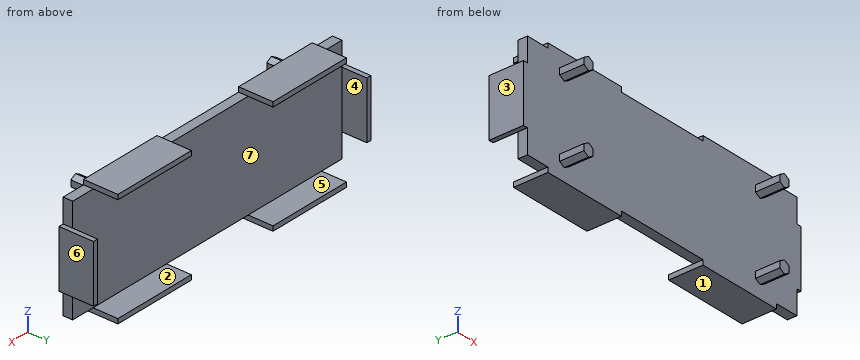
```python
from build123d import *

# Parameters (mm, degrees)
SKETCH1_W           = 165
SKETCH1_H           = 55
BOSS_EXTRUDE1_DEPTH = 5
SKETCH2_W           = 2.5
SKETCH2_H           = 30
BOSS_EXTRUDE2_DEPTH = 18
SKETCH3_W           = 45
SKETCH3_H           = 2.5
BOSS_EXTRUDE3_DEPTH = 18
BOSS_EXTRUDE4_DEPTH = 12.75


with BuildPart() as part:
    # Sketch1 → Boss-Extrude1 (new body)
    with BuildSketch(Plane(origin=(0, 0, 0), x_dir=(1, 0, 0), z_dir=(0, 1, 0))):
        with Locations((82.5, 27.5)):
            Rectangle(SKETCH1_W, SKETCH1_H)
    extrude(amount=BOSS_EXTRUDE1_DEPTH)

    # Sketch2 → Boss-Extrude2 (add)
    with BuildSketch(Plane(origin=(0, 0, 0), x_dir=(1, 0, 0), z_dir=(0, 1, 0))):
        with Locations((166.25, 27.5)):
            Rectangle(SKETCH2_W, SKETCH2_H)
        with Locations((-1.25, 27.5)):
            Rectangle(SKETCH2_W, SKETCH2_H)
    extrude(amount=BOSS_EXTRUDE2_DEPTH)

    # Sketch3 → Boss-Extrude3 (add)
    with BuildSketch(Plane(origin=(0, 0, 0), x_dir=(1, 0, 0), z_dir=(0, 1, 0))):
        with Locations((130, 56.25)):
            Rectangle(SKETCH3_W, SKETCH3_H)
        with Locations((35, 56.25)):
            Rectangle(SKETCH3_W, SKETCH3_H)
        with Locations((130, -1.25)):
            Rectangle(SKETCH3_W, SKETCH3_H)
        with Locations((35, -1.25)):
            Rectangle(SKETCH3_W, SKETCH3_H)
    extrude(amount=BOSS_EXTRUDE3_DEPTH)

    # Sketch4 → Boss-Extrude4 (add)
    with BuildSketch(Plane.XZ):
        Polygon((139.65, -5.854551733), (139.65, -9.145448267), (142.5, -10.790896534), (145.35, -9.145448267), (145.35, -5.854551733), (142.5, -4.209103466), align=None)
        Polygon((22.5, -10.790896534), (25.35, -9.145448267), (25.35, -5.854551733), (22.5, -4.209103466), (19.65, -5.854551733), (19.65, -9.145448267), align=None)
        Polygon((22.5, -50.790896534), (25.35, -49.145448267), (25.35, -45.854551733), (22.5, -44.209103466), (19.65, -45.854551733), (19.65, -49.145448267), align=None)
        Polygon((145.35, -49.145448267), (145.35, -45.854551733), (142.5, -44.209103466), (139.65, -45.854551733), (139.65, -49.145448267), (142.5, -50.790896534), align=None)
    extrude(amount=BOSS_EXTRUDE4_DEPTH)


solid = part.part
```
Part model, mm, in its own coordinate system. Face numbers are marked on the shaded views. A direction names the side the tool comes from. Give positions to 0.01 mm unless a question says otherwise; leave off trailing zeros. Order: outer loops, then holes, each group sorted by start corner. A loop starts at its lowest first (then second) coordinate and runs counter-clockwise, first axis right, second up. Notation, with made-up numbers: (53.5, 15) - (72.5, 15) arc R17 ccw to (72.5, 27) - close; hole circle Ø11 at (9, 70.5). An arc over 180 degrees is marked (long way). Use one line per item in the form item = value.
Item 1: Slice it at D-D on x = 52.5. Give the cut face in (y, z).
Solution:
outline = (0, -57.5) - (18, -57.5) - (18, -55) - (5, -55) - (5, 0) - (18, 0) - (18, 2.5) - (0, 2.5) - close
Item 2: Slice it at B-B on y = -6. Give the cut face in (x, z).
Solution:
outline = (19.65, -49.15) - (22.5, -50.79) - (25.35, -49.15) - (25.35, -45.85) - (22.5, -44.21) - (19.65, -45.85) - close; (19.65, -9.15) - (22.5, -10.79) - (25.35, -9.15) - (25.35, -5.85) - (22.5, -4.21) - (19.65, -5.85) - close; (139.65, -49.15) - (142.5, -50.79) - (145.35, -49.15) - (145.35, -45.85) - (142.5, -44.21) - (139.65, -45.85) - close; (139.65, -9.15) - (142.5, -10.79) - (145.35, -9.15) - (145.35, -5.85) - (142.5, -4.21) - (139.65, -5.85) - close
Item 3: Slice it at C-C on z = -25. Give the cut face in (x, y).
Solution:
outline = (-2.5, 0) - (167.5, 0) - (167.5, 18) - (165, 18) - (165, 5) - (0, 5) - (0, 18) - (-2.5, 18) - close
Item 4: Two-plate mould, pull along Z, no slides. Class the marked faces 1, 2 and 3: released by +Z, released by -Z, zero draft, split by the parting line, or undercut.
Solution:
face_1 = released by -Z
face_2 = undercut
face_3 = zero draft
Item 5: Slice it at A-A on y = 12. Give the cut face in (x, z).
Solution:
outline = (-2.5, -42.5) - (0, -42.5) - (0, -12.5) - (-2.5, -12.5) - close; (12.5, -57.5) - (57.5, -57.5) - (57.5, -55) - (12.5, -55) - close; (12.5, 0) - (57.5, 0) - (57.5, 2.5) - (12.5, 2.5) - close; (107.5, -57.5) - (152.5, -57.5) - (152.5, -55) - (107.5, -55) - close; (107.5, 0) - (152.5, 0) - (152.5, 2.5) - (107.5, 2.5) - close; (165, -42.5) - (167.5, -42.5) - (167.5, -12.5) - (165, -12.5) - close
Item 6: Pin check, flat tips, straight feed: pin 1 Ø10 at (y, z) = (0.5, -50.5) entering from +X; pin 2 Ø3 at (y, z) = (9.5, 1.5) entering from +X; pin 3 Ø1.5 at (x, y) = (157.5, 3) entering from +Z; pin 4 Ø12 at (y, z) = (-8, -29) entering from -X. Stop position of each tip, or through.
Solution:
pin_1 = 165
pin_2 = 152.5
pin_3 = 0
pin_4 = through
Item 7: Which spindle directions (+Z, -Z, +X, -X, +Y, -Y) get a long thin tool onto all of the face, cutting with end or side? Do the marked faces 4, 5, 6 and 7. Say none if no direction does.
Solution:
face_4 = +Z, -Z, +Y
face_5 = +X, -X, +Y
face_6 = +Z, -Z, +X, +Y, -Y
face_7 = +Y
Item 8: Probe probe 1 along X at (y, z) = (8.5, -23.5); probe 2 along X at (y, z) = (-7, -48); probe 3 along Z at (x, y) = (22.5, 8.5). List the from-to ranges inside material, lowest first. Write a range as from..to.
Solution:
probe_1 = -2.5..0, 165..167.5
probe_2 = 19.65..25.35, 139.65..145.35
probe_3 = -57.5..-55, 0..2.5
